Check sheet for the modelled part. Datum: model origin and axes. Units: mm. Round coordinates to 2 decimals unless told otherwise and drop trailing zeros. Loops run counter-clockwise (first coordinate to the right, second up) from the corner with the lowest first, then second, coordinate; pieces in that order, holes last. Notation, with made-up numbers: (22.25, 15.5) -> (36.25, 15.5) arc R16 ccw to (36.25, 44.5) -> close; hole circle Ø7 at (-37.75, 63.5). An arc over 180 degrees is marked (long way). Use one line per item in the form item = value. Start each with the question number.
(1) Sectioned sample at A-A (x = 3.5). Record the cut outline in (y, z), and give its area (3 significant figures).
(2) Go/stop test with flat-tipped pins: pin 1 (3 mm diameter, centred on y = 5.5, z = -178, fed in from +X); pin 2 (0.5 mm diameter, centred on x = 0.5, z = -262.5, fed in from +Y); pin 3 (0.5 mm diameter, centred on x = 0.5, z = -135.5, fed in from -Y). Record where each tip stops, or that it passes through.
(3) Material ranges on probe 1 along Y at (x, z) = (2.75, -316); probe 2 along Y at (x, z) = (0.75, -330); probe 3 along X at (y, z) = (10, -389), recorded low to high. Write a range as [from, to].
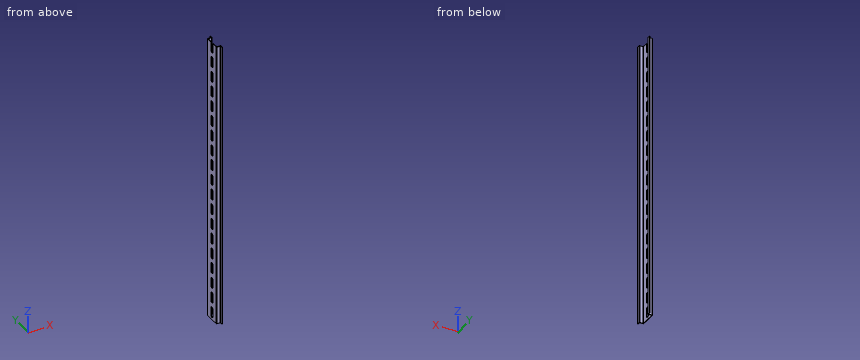
from build123d import *

# Parameters (mm, degrees)
BOSS_EXTRUDE1_DEPTH = 500
CUT_EXTRUDE1_DEPTH  = 7.5
LPATTERN1_COUNT     = 40
LPATTERN1_PITCH     = 25
SKETCH3_W           = 59.422885842
SKETCH3_H           = 88.158569076
CUT_EXTRUDE2_DEPTH  = 530


with BuildPart() as part:
    # Sketch1 → Boss-Extrude1 (new, symmetric)
    with BuildSketch(Plane.XY):
        with BuildLine():
            Line((7.5, 17.5), (6.5, 17.5))
            Line((6.5, 17.5), (6.5, 14))
            ThreePointArc((6.5, 14), (6.353553391, 13.646446609), (6, 13.5))
            Line((6, 13.5), (1, 13.5))
            ThreePointArc((1, 13.5), (0.292893219, 13.207106781), (0, 12.5))
            Line((0, 12.5), (0, -12.5))
            ThreePointArc((0, -12.5), (0.292893219, -13.207106781), (1, -13.5))
            Line((1, -13.5), (6, -13.5))
            ThreePointArc((6, -13.5), (6.353553391, -13.646446609), (6.5, -14))
            Line((6.5, -14), (6.5, -17.5))
            Line((6.5, -17.5), (7.5, -17.5))
            Line((7.5, -17.5), (7.5, -13.5))
            ThreePointArc((7.5, -13.5), (7.207106781, -12.792893219), (6.5, -12.5))
            Line((6.5, -12.5), (1.5, -12.5))
            ThreePointArc((1.5, -12.5), (1.146446609, -12.353553391), (1, -12))
            Line((1, -12), (1, 12))
            ThreePointArc((1, 12), (1.146446609, 12.353553391), (1.5, 12.5))
            Line((1.5, 12.5), (6.5, 12.5))
            ThreePointArc((6.5, 12.5), (7.207106781, 12.792893219), (7.5, 13.5))
            Line((7.5, 13.5), (7.5, 17.5))
        make_face()
    extrude(amount=BOSS_EXTRUDE1_DEPTH, both=True)

    # Sketch2 → Cut-Extrude1 (cut)
    with BuildSketch(Plane(origin=(0, 0, 0), x_dir=(0, 0, -1), z_dir=(1, 0, 0))):
        with BuildLine():
            Line((-493.35, 3.15), (-481.65, 3.15))
            ThreePointArc((-481.65, 3.15), (-478.5, 0), (-481.65, -3.15))
            Line((-481.65, -3.15), (-493.35, -3.15))
            ThreePointArc((-493.35, -3.15), (-496.5, 0), (-493.35, 3.15))
        make_face()
    cut_extrude1 = extrude(amount=CUT_EXTRUDE1_DEPTH, mode=Mode.SUBTRACT)

    # LPattern1: Cut-Extrude1 ×40
    with Locations(*[(0, 0, -i * LPATTERN1_PITCH) for i in range(1, LPATTERN1_COUNT)]):
        add(cut_extrude1, mode=Mode.SUBTRACT)

    # Sketch3 → Cut-Extrude2 (cut)
    with BuildSketch(Plane.XY.offset(500)):
        Rectangle(SKETCH3_W, SKETCH3_H)
    extrude(amount=-CUT_EXTRUDE2_DEPTH, mode=Mode.SUBTRACT)


solid = part.part
Checks:
q1.outline = (-13.5, -500) -> (-12.5, -500) -> (-12.5, -30) -> (-13.5, -30) -> close; (12.5, -500) -> (13.5, -500) -> (13.5, -30) -> (12.5, -30) -> close
q1.area = 940 mm2
q2.pin_1 = 1
q2.pin_2 = 13.47
q2.pin_3 = -13.47
q3.probe_1 = [-13.5, -12.5], [12.5, 13.5]
q3.probe_2 = [-13.47, -2.68], [2.68, 13.47]
q3.probe_3 = [0, 1]
